For this review, use the dimensioned drawing (mm, ordinates from the lowest corner) and the shaded views. A direction names the side the tool comes from. Coordinates: 2 decimals unless noted, no trailing zeros. Write each loop counter-clockwise with the first axis right and the second up, starting at its lowest first coordinate (ties: lowest second). Pieces come first, ordered by that corner, then holes. Notation, with made-up numbers: M 21.25,81.25 L 77.25,81.25 A19 ccw 77.25,97.25 Z; hole C 79.25,40.25 d10. An arc over 180 degrees is marked long. One line per question, with ' | ' between items.
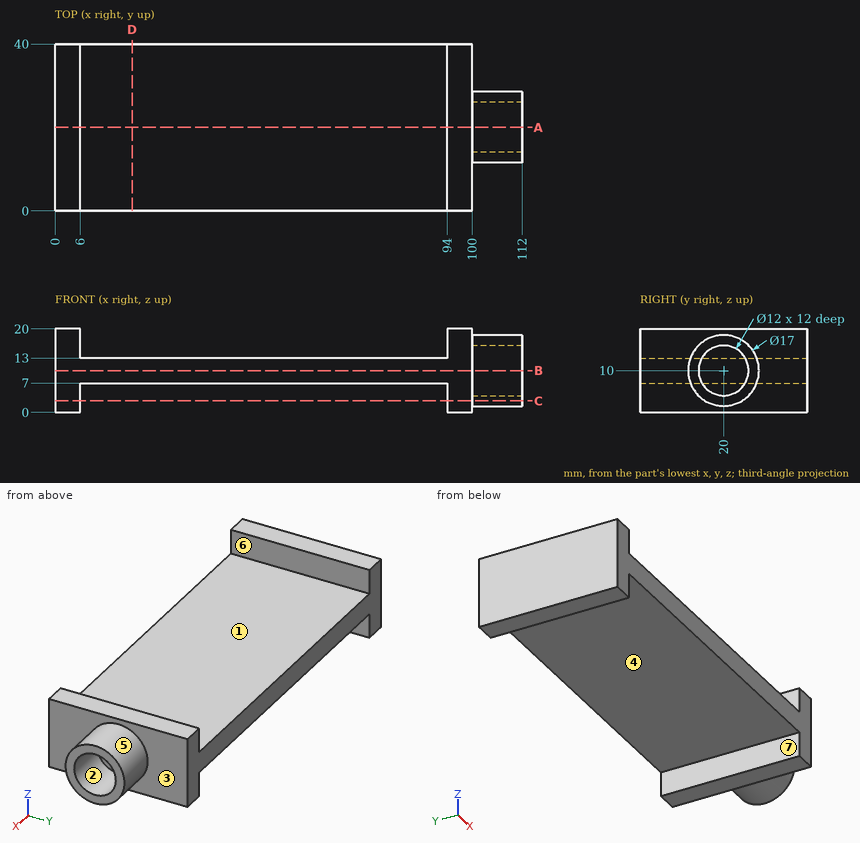
1. Take a section at D-D (x = 18.5). Write out the cut boundary in (y, z).
Answer sheet:
outline: M 0,7 L 40,7 L 40,13 L 0,13 Z
2. Insertion check: pin 1 Ø9.5 at (y, z) = (20, 10) entering from +X; pin 2 Ø4 at (x, y) = (12, 9) entering from -Z; pin 3 Ø20 at (x, y) = (29.5, 26.5) entering from +Z. Each pin has a flat end and moves straight along its axis. Give the tip position at first contact, or say it passes through.
Answer sheet:
pin 1: x = 100 | pin 2: z = 7 | pin 3: z = 13
3. Draft analysis for pull direction X (two halves, no side actions). For the marked faces 1, 2, 3 and 4, state which applies: pulls with the +X half, pulls with the -X half, needs draft (parallel to the pull), parting line crosses it, or undercut.
Answer sheet:
face 1: undercut | face 2: needs draft | face 3: pulls with the +X half | face 4: undercut
4. Take a section at A-A (y = 20). Write out the cut boundary in (x, z).
Answer sheet:
outline: M 0,0 L 6,0 L 6,7 L 94,7 L 94,0 L 100,0 L 100,1.5 L 112,1.5 L 112,4 L 100,4 L 100,16 L 112,16 L 112,18.5 L 100,18.5 L 100,20 L 94,20 L 94,13 L 6,13 L 6,20 L 0,20 Z
5. Tool access review of the marked faces 5, 6 and 7: name each direction out of +Z, -Z, +X, -X, +Y, -Y from which nothing blocks a thin tool from reaching the whole face with its end or side.
Answer sheet:
face 5: +X | face 6: +Z, +Y, -Y | face 7: -Z, +Y, -Y
6. To check wall thickness, follow line 1 along Y through (x, z) = (109, 10); line 2 along X through (y, z) = (5, 14.25); line 3 along X through (y, z) = (17.5, 17). State the ranges of each line that lie inside material, in increasing order. Write a range as [from, to].
Answer sheet:
line 1: [11.5, 14], [26, 28.5] | line 2: [0, 6], [94, 100] | line 3: [0, 6], [94, 112]
7. Take a section at B-B (z = 10). Write out the cut boundary in (x, y).
Answer sheet:
outline: M 0,0 L 100,0 L 100,11.5 L 112,11.5 L 112,14 L 100,14 L 100,26 L 112,26 L 112,28.5 L 100,28.5 L 100,40 L 0,40 Z
8. Take a section at C-C (z = 2.75). Write out the cut boundary in (x, y).
Answer sheet:
outline: M 0,0 L 6,0 L 6,40 L 0,40 Z; M 94,0 L 100,0 L 100,15.56 L 112,15.56 L 112,24.44 L 100,24.44 L 100,40 L 94,40 Z
